Design review of the part built by this model. Coordinates are the model's own, in mm. A direction names the side the tool comes from. Round coordinates to 2 decimals unless told otherwise and drop trailing zeros. Write each loop counter-clockwise with the first axis right and the second up, starting at its lowest first coordinate (ties: lowest second). Pieces come first, ordered by that corner, then holes. Notation, with made-up numbers: M -22,11 L -4,11 A23 cw -4,34 Z; hole C 50.25,-28 d8. An arc over 180 degrees is marked long. One line per question, with ' | ' between items. Start each with the question number.
Item 1: Insertion check: pin 1 Ø1 at (y, z) = (12.5, 1) entering from -X; pin 2 Ø3 at (x, y) = (0.5, -23) entering from +Z; pin 3 Ø1.5 at (y, z) = (-13.5, 1.5) entering from -X; pin 4 Ø4 at (x, y) = (0, 25) entering from -Z. Each pin has a flat end and moves straight along its axis. Give the tip position at first contact, or say it passes through.
Item 2: For L1, parallel to Y at x = 0, z = 1.4 (3 decimals); L2, parallel to Y at x = 0, z = 5.1 (3 decimals); L3, parallel to X at y = -2.5, z = 1.4, list the stretches that pass through material, from the lowest coordinate up.
Item 3: Machinability: for faces 1 (the face through (19.78, 0.23, 4.03)), 2 (the face through (0, 0, 0)), which of the approach directions +Z, -Z, +X, -X, +Y, -Y give a long, thin tool a straight path to every point of the face, cutting with its end or side? Answer none if there is none.
Item 4: Add section A-A, the plane y = 0. State the section outline as (x, z) points (3 decimals).
Item 5: Add section C-C, the plane y = 23. State the section outline as (x, z) points.
Item 6: Add section D-D, the plane z = 1.2. State the section outline as (x, y) points (3 decimals).
Item 7: Draft analysis for pull direction Y (two halves, no side actions). For faces 3 (the face through (0, 0, 6)), 4 (the face through (-30.22, 0.23, 4.03)), 5 (the face through (-4.101, 31.232, 2.958)), state which applies: released by +Y, released by -Y, zero draft, split by the parting line, or undercut.
```python
from build123d import *

# Parameters (mm, degrees)
SKETCH1_R              = 31.5
SKETCH1_R_2            = 3.225
MAIN_PA10_FLANGE_DEPTH = 6
SKETCH3_R              = 5.225
M6_HOLE_DEPTH          = 4


with BuildPart() as part:
    # Sketch1 → Main PA10 Flange (new body)
    with BuildSketch(Plane.XY):
        Circle(SKETCH1_R)
        with Locations((0, -25)):
            Circle(SKETCH1_R_2, mode=Mode.SUBTRACT)
        with Locations((-25, 0)):
            Circle(SKETCH1_R_2, mode=Mode.SUBTRACT)
        with Locations((0, 25)):
            Circle(SKETCH1_R_2, mode=Mode.SUBTRACT)
        with Locations((25, 0)):
            Circle(SKETCH1_R_2, mode=Mode.SUBTRACT)
    extrude(amount=MAIN_PA10_FLANGE_DEPTH)

    # Sketch3 → M6 Hole (cut)
    with BuildSketch(Plane.XY.offset(6)):
        with Locations((0, -25)):
            Circle(SKETCH3_R)
        with Locations((-25, 0)):
            Circle(SKETCH3_R)
        with Locations((0, 25)):
            Circle(SKETCH3_R)
        with Locations((25, 0)):
            Circle(SKETCH3_R)
    extrude(amount=-M6_HOLE_DEPTH, mode=Mode.SUBTRACT)


solid = part.part
```
Computed values:
1) pin 1: stops at x = -29.12 | pin 2: stops at z = 2 | pin 3: stops at x = -28.8 | pin 4: passes through
2) L1: y = -31.5 to -28.225, -21.775 to 21.775, 28.225 to 31.5 | L2: y = -31.5 to -30.225, -19.775 to 19.775, 30.225 to 31.5 | L3: x = -31.4 to -27.04, -22.96 to 22.96, 27.04 to 31.4
3) face 1: +Z | face 2: -Z, +X, -X, +Y, -Y
4) outline: M -31.5,0 L -28.225,0 L -28.225,2 L -30.225,2 L -30.225,6 L -31.5,6 Z; M -21.775,0 L 21.775,0 L 21.775,2 L 19.775,2 L 19.775,6 L -19.775,6 L -19.775,2 L -21.775,2 Z; M 28.225,0 L 31.5,0 L 31.5,6 L 30.225,6 L 30.225,2 L 28.225,2 Z
5) outline: M -21.52,0 L -2.53,0 L -2.53,2 L -4.83,2 L -4.83,6 L -21.52,6 Z; M 2.53,0 L 21.52,0 L 21.52,6 L 4.83,6 L 4.83,2 L 2.53,2 Z
6) outline: C 0,0 d63; hole C -25,0 d6.45; hole C 0,-25 d6.45; hole C 0,25 d6.45; hole C 25,0 d6.45
7) face 3: zero draft | face 4: undercut | face 5: split by the parting line
